from build123d import *

# Parameters (mm, degrees)
SKETCH_1_R          = 5
SKETCH_1_R_2        = 3.1
EXTRUDE_1_DEPTH     = 4
SKETCH_1_3_R        = 20
SKETCH_1_3_R_2      = 18
EXTRUDE_2_DEPTH     = 4
SKETCH_1_4_R        = 20
SKETCH_1_4_R_2      = 18
SKETCH_1_4_R_3      = 5
SKETCH_1_4_R_4      = 3.1
EXTRUDE_3_DEPTH     = 2
SKETCH_2_R          = 20
EXTRUDE_4_DEPTH     = 1.8
SKETCH_4_R          = 18
SKETCH_4_R_2        = 5
CUT_EXTRUDE_1_DEPTH = 1.8


with BuildPart() as part:
    # Sketch 1 → Extrude 1 (new body)
    with BuildSketch(Plane.XY):
        Circle(SKETCH_1_R)
        Circle(SKETCH_1_R_2, mode=Mode.SUBTRACT)
    extrude(amount=EXTRUDE_1_DEPTH)



with BuildPart() as body_2:
    # Sketch 1_3 → Extrude 2 (new body)
    with BuildSketch(Plane.XY):
        Circle(SKETCH_1_3_R)
        Circle(SKETCH_1_3_R_2, mode=Mode.SUBTRACT)
    extrude(amount=EXTRUDE_2_DEPTH)


with BuildPart() as part_1:
    add(part.part)

    add(body_2.part)  # Extrude 3 merges body 2
    # Sketch 1_4 → Extrude 3 (add)
    with BuildSketch(Plane.XY):
        Circle(SKETCH_1_4_R)
        Circle(SKETCH_1_4_R_2, mode=Mode.SUBTRACT)
        Circle(SKETCH_1_4_R_2)
        Circle(SKETCH_1_4_R_3, mode=Mode.SUBTRACT)
        Circle(SKETCH_1_4_R_3)
        Circle(SKETCH_1_4_R_4, mode=Mode.SUBTRACT)
        Circle(SKETCH_1_4_R_4)
    extrude(amount=-EXTRUDE_3_DEPTH)

    # Sketch 2 → Extrude 4 (add)
    with BuildSketch(Plane(origin=(0, 0, -2), x_dir=(-1, 0, 0), z_dir=(0, 0, -1))):
        with Locations(Location((0, 0, 0), (0, 0, 180))):
            Circle(SKETCH_2_R)
    extrude(amount=EXTRUDE_4_DEPTH)

    # Sketch 4 → Cut-Extrude 1 (cut)
    with BuildSketch(Plane.XY):
        Circle(SKETCH_4_R)
        Circle(SKETCH_4_R_2, mode=Mode.SUBTRACT)
    extrude(amount=-CUT_EXTRUDE_1_DEPTH, mode=Mode.SUBTRACT)


solid = part_1.part
Work out the finished part from the listing and answer in its coordinate system (mm). A direction names the side the tool comes from. Coordinates: 2 decimals unless noted, no trailing zeros. Order: outer loops, then holes, each group sorted by start corner. A loop starts at its lowest first (then second) coordinate and runs counter-clockwise, first axis right, second up. Notation, with made-up numbers: (54, 78.5) - (70, 78.5) arc R33 cw to (70, 117.5) - close; hole circle Ø4 at (45.5, 24). An arc over 180 degrees is marked (long way). Put each result on its own line as item: value. Start each with the question number.
1) Find the intervals of material crossed by line 1 (Y direction, x = 0, z = 2.55); line 2 (Y direction, x = 0, z = -0.5); line 3 (Y direction, x = 4.5, z = 0), in increasing order. Write a range as from..to.
2) For faces 1 (the flat face through (-0.1, -3.3, 4)), 2 (the flat face through (4, -4, -1.8)), determine the directions among +Z, -Z, +X, -X, +Y, -Y from which every point of the face is accessible in a straight line to the end or side of a thin tool.
3) Flat-ended cylindrical pins translate along their axes: pin 1 (1.5 mm diameter, centred on x = -16, z = 1.5, fed in from +Y); pin 2 (1.9 mm diameter, centred on x = -1, y = 0.5, fed in from +Z); pin 3 (1 mm diameter, centred on x = -15, y = 1, fed in from +Z). Find the tip coordinate at first contact, or state that the pin passes through.
4) Find section D-D (z = 2). Give the vertices of the cut face in (x, y), plus the area to 3 significant figures.
5) Find section A-A (z = -1.25). Give the vertices of the cut face in (x, y).
6) Find section B-B (x = 0). Give the vertices of the cut face in (y, z), plus the area to 3 significant figures.
7) For a pull along X with two mould halves and no side action, classify faces 3 (the cylindrical face through (1.43, -2.75, 1.97)), 4 (the flat face through (0, 0, -3.8)) as released by +X, released by -X, zero draft, split by the parting line, or undercut.
Results list:
1. line 1: y = -20..-18, -5..-3.1, 3.1..5, 18..20
1. line 2: y = -20..-18, -5..5, 18..20
1. line 3: y = -19.49..-17.43, -2.18..2.18, 17.43..19.49
2. face 1: +Z, +X, -X, +Y, -Y
2. face 2: +Z
3. pin 1: stops at y = 12.94
3. pin 2: stops at z = 0
3. pin 3: stops at z = -1.8
4. outline: circle Ø40 at (0, 0); circle Ø10 at (0, 0); hole circle Ø36 at (0, 0); hole circle Ø6.2 at (0, 0)
4. area: 287 mm^2
5. outline: circle Ø40 at (0, 0); circle Ø10 at (0, 0); hole circle Ø36 at (0, 0)
6. outline: (-20, -3.8) - (20, -3.8) - (20, 4) - (18, 4) - (18, -1.8) - (5, -1.8) - (5, 4) - (3.1, 4) - (3.1, 0) - (-3.1, 0) - (-3.1, 4) - (-5, 4) - (-5, -1.8) - (-18, -1.8) - (-18, 4) - (-20, 4) - close
6. area: 136 mm^2
7. face 3: undercut
7. face 4: zero draft
